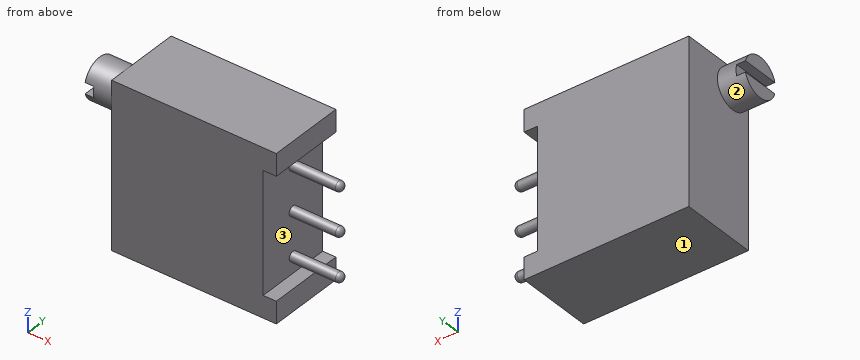
Autodesk Inventor part; units mm, degrees
ref_plane "YZ Plane" through (0, 0, 0) normal (1, 0, 0) x (0, 1, 0)
ref_plane "XZ Plane" through (0, 0, 0) normal (0, 1, 0) x (-1, 0, 0)
ref_plane "XY Plane" through (0, 0, 0) normal (0, 0, 1) x (1, 0, 0)
sketch "Sketch1" plane through (0, 0, 0) normal (0, 1, 0) x (-1, 0, 0)
  line L0 (0, 0) -> (9.525, 0)
  line L1 (9.525, 0) -> (9.525, -9.525)
  line L2 (9.525, -9.525) -> (0, -9.525)
  line L3 (0, -9.525) -> (0, -8.255)
  line L4 (0, -8.255) -> (0.762, -8.255)
  line L5 (0.762, -8.255) -> (0.762, -1.27)
  line L6 (0.762, -1.27) -> (0, -1.27)
  line L7 (0, -1.27) -> (0, 0)
  dimension "d0" = 9.525
  dimension "d1" = 9.525
  dimension "d2" = 6.985
  dimension "d3" = 0.762
extrude "Extrusion1" add sketch "Sketch1" along normal blind 4.445
sketch "Sketch2" plane through (-0.762, 0, -1.27) normal (1, 0, 0) x (0, 0, -1)
  circle A0 centre (3.4925, 2.2225) radius 0.2794
  circle A1 centre (0.9525, 2.2225) radius 0.2794
  circle A2 centre (6.0325, 2.2225) radius 0.2794
  line L0 (0, 4.445) -> (6.985, 4.445) construction
  line L1 (0, 0) -> (0, 4.445) construction
  point P0 (-1.27, 0)
  point P1 (3.4925, 4.445)
  point P2 (0, 2.2225)
  dimension "d6" = 0.5588
  dimension "d7" = 2.54
  dimension "d8" = 2.54
extrude "Extrusion2" add sketch "Sketch2" along normal blind 2.921
sketch "Sketch3" plane through (-9.525, 0, -9.525) normal (-1, 0, 0) x (0, 0, 1)
  circle A0 centre (8.3566, 1.1684) radius 1.143
  line L0 (9.525, 0) -> (0, 0)
  line L1 (9.525, 0) -> (9.525, 4.445)
  dimension "d11" = 2.286
  dimension "d12" = 1.1684
  dimension "d13" = 1.1684
extrude "Extrusion3" add sketch "Sketch3" along normal blind 1.5875
sketch "Sketch4" plane through (0, 0, 0) normal (0, -1, 0) x (1, 0, 0)
  line L0 (-11.1125, -1.4859) -> (-10.6045, -1.4859)
  line L1 (-10.6045, -1.4859) -> (-10.6045, -0.8509)
  line L2 (-10.6045, -0.8509) -> (-11.1125, -0.8509)
  line L3 (-11.1125, -0.8509) -> (-11.1125, -1.4859)
  line L4 (-11.1125, -0.0254) -> (-11.1125, -2.3114)
  point P0 (0, 0)
  point P1 (-11.1125, -1.1684)
  dimension "d16" = 0.508
  dimension "d17" = 0.635
extrude "Extrusion4" cut sketch "Sketch4" against normal through all
fillet "Fillet1" radius 0.254 3 edges at (2.159, 2.2225, -7.0231) (2.159, 2.2225, -4.4831) (2.159, 2.2225, -1.9431)
equation "\"d8\" = d7"
equation "\"d13\" = d12"
properties part number "Precision Trim Pot - baoter 3296"
Can you work these out from the model? Positions are in its coordinate system, mm. Face numbers are marked on the shaded views. A direction names the side the tool comes from. Give positions to 0.01 mm unless a question says otherwise; leave off trailing zeros. Write each loop counter-clockwise with the first axis right and the second up, starting at its lowest first coordinate (ties: lowest second). Pieces come first, ordered by that corner, then holes. Notation, with made-up numbers: (4.5, 37) -> (25.5, 37) arc R26 cw to (25.5, 67) -> close; hole circle Ø8 at (19, 67). An arc over 180 degrees is marked (long way). One line per item, written item: value.
Q1. Which directions (+Z, -Z, +X, -X, +Y, -Y) give clear straight access to the entire face, cutting with the end or side of a thin tool? Please do the marked faces 1, 2 and 3.
Results found:
face 1: -Z, +X, -X, +Y, -Y
face 2: -X
face 3: +X
Q2. For P1, Ø1, axis at y = 2.5, z = -8.5, coming from the +X side; P2, Ø0.6, axis at x = -11, y = 0.5, coming from the -Z side; P3, Ø1.3, axis at y = 3, z = -5, coming from the -X side (3 decimals), each with a flat end and sliding along its axis, tell me the tip position at first contact or that it passes through.
Results found:
P1: stops at x = 0
P2: stops at z = -2.25
P3: stops at x = -9.525
Q3. Imagine slicing it at B-B on z = -3.25. Please give me the cut outline in (x, y) (3 decimals), and give its area (3 significant figures).
Results found:
outline: (-9.525, 0) -> (-0.762, 0) -> (-0.762, 4.445) -> (-9.525, 4.445) -> close
area: 39.0 mm^2
Q4. Imagine slicing it at D-D on x = -9.75. Please give me the cut outline in (y, z).
Results found:
outline: circle Ø2.29 at (1.17, -1.17)
Q5. Please list where these lines run through material, in increasing order: line 1 (Z direction, x = -0.25, y = 2.05) (3 decimals); line 2 (X direction, y = 3.5, z = -6.5) (3 decimals); line 3 (X direction, y = 0.45, z = -8.75) (3 decimals). Write a range as [from, to].
Results found:
line 1: z = [-9.525, -8.255], [-7.522, -7.083], [-4.982, -4.543], [-2.442, -2.003], [-1.27, 0]
line 2: x = [-9.525, -0.762]
line 3: x = [-9.525, 0]
Q6. Imagine slicing it at A-A on y = 2.9. Please give me the cut outline in (x, z) (3 decimals), and give its area (3 significant figures).
Results found:
outline: (-9.525, -9.525) -> (0, -9.525) -> (0, -8.255) -> (-0.762, -8.255) -> (-0.762, -1.27) -> (0, -1.27) -> (0, 0) -> (-9.525, 0) -> close
area: 85.4 mm^2
